from build123d import *

# Parameters (mm, degrees)
SKETCH1_W           = 12
SKETCH1_H           = 32.5
SKETCH1_R           = 1
SKETCH1_W_2         = 6
SKETCH1_H_2         = 12.9
BOSS_EXTRUDE1_DEPTH = 3.5
FILLET1_R           = 1.2
FILLET2_R           = 6
SKETCH2_R           = 5.2
SKETCH2_R_2         = 3.7
BOSS_EXTRUDE2_DEPTH = 2.5


with BuildPart() as part:
    # Sketch1 → Boss-Extrude1 (new body)
    with BuildSketch(Plane.XY.offset(10)):
        with Locations((-276.988860295, 267.101135254)):
            Rectangle(SKETCH1_W, SKETCH1_H)
        with Locations((-281.069234982, 280.854420413)):
            Circle(SKETCH1_R, mode=Mode.SUBTRACT)
        with Locations((-273.069234982, 280.854420413)):
            Circle(SKETCH1_R, mode=Mode.SUBTRACT)
        with Locations((-276.994472892, 271.487209026)):
            Rectangle(SKETCH1_W_2, SKETCH1_H_2, mode=Mode.SUBTRACT)
    extrude(amount=BOSS_EXTRUDE1_DEPTH)

    # Fillet1
    fillet1_edges = [part.edges().sort_by_distance(p)[0] for p in [
        (-279.994472892, 277.937209026, 11.75),
        (-279.994472892, 265.037209026, 11.75),
        (-273.994472892, 265.037209026, 11.75),
        (-273.994472892, 277.937209026, 11.75),
        (-282.988860295, 283.351135254, 11.75),
        (-270.988860295, 283.351135254, 11.75),
    ]]
    fillet(fillet1_edges, radius=FILLET1_R)

    # Fillet2
    fillet2_edges = [part.edges().sort_by_distance(p)[0] for p in [
        (-282.988860295, 250.851135254, 11.75),
        (-270.988860295, 250.851135254, 11.75),
    ]]
    fillet(fillet2_edges, radius=FILLET2_R - 0.0001)  # a hair under: the kernel refuses the full size

    # Sketch2 → Boss-Extrude2 (add)
    with BuildSketch(Plane.XY.offset(13.5)):
        with Locations((-277.110164077, 256.96399239)):
            Circle(SKETCH2_R)
        with Locations((-277.110164077, 256.96399239)):
            Circle(SKETCH2_R_2, mode=Mode.SUBTRACT)
    extrude(amount=BOSS_EXTRUDE2_DEPTH)


solid = part.part
Can you work these out from the model? Positions are in its coordinate system, mm. A direction names the side the tool comes from. Coordinates: 2 decimals unless noted, no trailing zeros. Write each loop counter-clockwise with the first axis right and the second up, starting at its lowest first coordinate (ties: lowest second). Pieces come first, ordered by that corner, then holes. Notation, with made-up numbers: (86, 67.5) - (97, 67.5) arc R11 ccw to (97, 73.5) - close; hole circle Ø5 at (70, -18). An arc over 180 degrees is marked (long way). Return JSON: item names as keys, results as strings. Group by question number.
Item 1: If we section it at A-A (y = 275): Write out the boundary of the cut face in (x, z), then the cut area to 3 significant figures.
Item 2: We'd pull the mould along X, two halves only. Please class faces 1 (the face through (-277, 257, 13.5)), 2 (the face through (-277, 264, 10)), 3 (the face through (-274.71, 252.35, 14.73)), 4 (the face through (-274.355, 265.379, 11.774)): pulls with the +X half, pulls with the -X half, needs draft (parallel to the pull), parting line crosses it, or undercut.
Item 3: If we section it at C-C (z = 11.35): Count the separate pieces of the cut face and the enclosed holes in it, then the cut area to 3 significant figures.
Item 4: I'm going to push flat-ended pins straight in: pin 1 Ø2 at (x, y) = (-277.5, 257.5) entering from +Z; pin 2 Ø3 at (x, y) = (-273.07, 280.85) entering from -Z; pin 3 Ø1 at (x, z) = (-275.5, 14.5) entering from -Y. Where does each tip first touch, or does it pass through?
Item 5: Please list where these lines run through material, in increasing order: probe 1 along X at (y, z) = (272, 11.05); probe 2 along Y at (x, z) = (-277.25, 10.5); probe 3 along Z at (x, y) = (-276.75, 265).
Item 6: If we section it at D-D (y = 258.5): Write out the boundary of the cut face in (x, z), then the cut area to 3 significant figures.
Item 7: Which directions (+Z, -Z, +X, -X, +Y, -Y) give clear straight access to the entire face, cutting with the end or side of a thin tool? Please do faces 5 (the face through (-279.634, 265.379, 11.774)), 6 (the face through (-279.84, 259.46, 14.73)), 7 (the face through (-282.989, 269, 12)).
Item 8: If we section it at B-B (x = -280.5): Write out the boundary of the cut face in (y, z).
Return value:
{
 "1": {"outline": "(-282.99, 10) - (-279.99, 10) - (-279.99, 13.5) - (-282.99, 13.5) - close; (-273.99, 10) - (-270.99, 10) - (-270.99, 13.5) - (-273.99, 13.5) - close", "area": "21.0 mm^2"},
 "2": {"face 1": "undercut", "face 2": "needs draft", "face 3": "parting line crosses it", "face 4": "undercut"},
 "3": {"separate pieces": "1", "enclosed holes": "3", "area": "291 mm^2"},
 "4": {"pin 1": "stops at z = 13.5", "pin 2": "stops at z = 10", "pin 3": "stops at y = 251.88"},
 "5": {"probe 1": "x = -282.99 to -279.99, -273.99 to -270.99", "probe 2": "y = 250.86 to 265.04, 277.94 to 283.35", "probe 3": "z = 10 to 13.5"},
 "6": {"outline": "(-282.99, 10) - (-270.99, 10) - (-270.99, 13.5) - (-272.14, 13.5) - (-272.14, 16) - (-273.74, 16) - (-273.74, 13.5) - (-280.48, 13.5) - (-280.48, 16) - (-282.08, 16) - (-282.08, 13.5) - (-282.99, 13.5) - close", "area": "50.0 mm^2"},
 "7": {"face 5": "+Z, -Z", "face 6": "+Z", "face 7": "+Z, -Z, -X, +Y, -Y"},
 "8": {"outline": "(251.99, 10) - (280.03, 10) - (280.03, 13.5) - (260.91, 13.5) - (260.91, 16) - (258.45, 16) - (258.45, 13.5) - (255.48, 13.5) - (255.48, 16) - (253.02, 16) - (253.02, 13.5) - (251.99, 13.5) - close; (281.68, 10) - (283.35, 10) - (283.35, 13.5) - (281.68, 13.5) - close"}
}
